```python
from build123d import *

# Parameters (mm, degrees)
BOSS_EXTRUDE1_DEPTH      = 48
BOSS_EXTRUDE2_DEPTH      = 107
BOSS_EXTRUDE2_DEPTH_BACK = 135
BOSS_EXTRUDE3_DEPTH      = 70


with BuildPart() as part:
    # Sketch6 → Boss-Extrude1 (new body)
    with BuildSketch(Plane.YZ):
        with BuildLine():
            Line((-18.5, 42), (9, 42))
            Line((9, 42), (9, -20))
            ThreePointArc((9, -20), (6.656854249, -25.656854249), (1, -28))
            Line((1, -28), (-10.5, -28))
            ThreePointArc((-10.5, -28), (-16.156854249, -25.656854249), (-18.5, -20))
            Line((-18.5, -20), (-18.5, 42))
        make_face()
    extrude(amount=-BOSS_EXTRUDE1_DEPTH)

    # Sketch7 → Boss-Extrude2 (add, two sides: drawn at the far end of the back side and taken through both)
    with BuildSketch(Plane.YZ.offset(-BOSS_EXTRUDE2_DEPTH_BACK)):
        with BuildLine():
            Line((6.7, 42), (6.7, 0))
            ThreePointArc((6.7, 0), (0, -6.7), (-6.7, 0))
            Line((-6.7, 0), (-6.7, 42))
            Line((-6.7, 42), (6.7, 42))
        make_face()
    extrude(amount=BOSS_EXTRUDE2_DEPTH + BOSS_EXTRUDE2_DEPTH_BACK)

    # Sketch8 → Boss-Extrude3 (add)
    with BuildSketch(Plane.YZ):
        with BuildLine():
            Line((-17.499999986, -6.99976205), (-19.468374717, 42))
            Line((-19.468374717, 42), (-11.531625283, 42))
            Line((-11.531625283, 42), (-13.500019034, -7.008725467))
            ThreePointArc((-13.500019034, -7.008725467), (-15.504481719, -8.999994979), (-17.499999986, -6.99976205))
        make_face()
    extrude(amount=BOSS_EXTRUDE3_DEPTH)

    # Loft2: read off the stored shape, not the designer's step
    # Loft2: loft between two sections, ruled curve by curve
    loft2_from = [
        Edge.make_bspline([(-43, -12.5, 42), (-43, -12.5, 36.250008881), (-43, -12.5, 24.641436529), (-43, -12.5, 7.145431099), (-43, -12.5, -10.177895331), (-43, -12.5, -21.457402798), (-43, -12.5, -27.496400477), (-43, -12.735353866, -28.366169962), (-43, -13.470979996, -29.306081404), (-43, -14.433479869, -29.873432167), (-43, -15.500002282, -30.063307511), (-43, -16.566524261, -29.873430596), (-43, -17.529022849, -29.306078761), (-43, -18.264647219, -28.36616736), (-43, -18.5, -27.496399176), (-43, -18.5, -21.457400197), (-43, -18.5, -10.177897954), (-43, -18.5, 7.145406937), (-43, -18.5, 24.641401673), (-43, -18.5, 36.249991119), (-43, -18.5, 42)], [0, 0, 0, 0, 0.114724944, 0.229449887, 0.344174831, 0.458899774, 0.458899774, 0.469174653, 0.479449533, 0.489724412, 0.499999291, 0.51027417, 0.52054905, 0.530823929, 0.541098808, 0.541098808, 0.655824106, 0.770549404, 0.885274702, 1, 1, 1, 1], 3),
        Edge.make_line((-43, -18.5, 42), (-43, -12.5, 42)),
    ]
    loft2_to = [
        Edge.make_bspline([(-90, -11.531625283, 42), (-90, -11.570656574, 37.916659954), (-90, -11.648004314, 29.824764413), (-90, -11.763499254, 17.742019914), (-90, -11.880008186, 5.553194479), (-90, -11.95947034, -2.759904881), (-90, -12, -7.379764452), (-90, -12.124025603, -8.182036975), (-90, -12.791211148, -9.362294599), (-90, -13.96862904, -10.268779081), (-90, -15.499994859, -10.616349391), (-90, -17.031362783, -10.268783245), (-90, -18.208784945, -9.362299724), (-90, -18.87597374, -8.182040057), (-90, -19, -7.379765435), (-90, -18.956733754, -2.759907847), (-90, -18.871906161, 5.553196207), (-90, -18.747530231, 17.742037363), (-90, -18.624236843, 29.824789377), (-90, -18.541666598, 37.916673379), (-90, -18.5, 42)], [0, 0, 0, 0, 0.114724944, 0.229449887, 0.344174831, 0.458899774, 0.458899774, 0.469174653, 0.479449533, 0.489724412, 0.499999291, 0.51027417, 0.52054905, 0.530823929, 0.541098808, 0.541098808, 0.655824106, 0.770549404, 0.885274702, 1, 1, 1, 1], 3),
        Edge.make_line((-90, -18.5, 42), (-90, -11.531625283, 42)),
    ]
    loft2 = Solid(Shell([*[Face.make_surface_from_curves(loft2_from[k], loft2_to[k]) for k in range(2)], Face(Wire(loft2_from)), Face(Wire(loft2_to))]))
    add(loft2)


solid = part.part
```
For this review, take the finished solid that the model builds, in its own axes (mm). A direction names the side the tool comes from. Coordinates: 2 decimals unless noted, no trailing zeros. Order: outer loops, then holes, each group sorted by start corner. A loop starts at its lowest first (then second) coordinate and runs counter-clockwise, first axis right, second up. Notation, with made-up numbers: (-26, 20) -> (1, 20) arc R30 ccw to (1, 59) -> close; hole circle Ø10 at (-34, 5). An arc over 180 degrees is marked (long way). Use CSV: the item, a comma, the result in double quotes. Start each with the question number.
Item 1: We need section A-A, the plane y = -3.25. Give the boundary of the cut face in (x, z), then the cut area to 3 significant figures.
Item 2: Wall thickness on probe 1 along Y at (x, z) = (1, 17); probe 2 along Y at (x, z) = (-110, 20); probe 3 along X at (y, z) = (-9.25, -4): over which ranges is each line inside the solid? List them lowest first.
Item 3: For faces 1 (the face through (0, -8, 0)), 2 (the face through (-92.1, 0.1, -6.7)), 3 (the face through (-90, -15, 16)), 4 (the face through (70, -15, 23)), 5 (the face through (34.51, -18.47, 17.16)), list the 3-axis set-ups (+Z, -Z, +X, -X, +Y, -Y) from which the entire face can be reached by the end or side of a thin tool; tool diameter is ignored.
Item 4: Draft analysis for pull direction Y (two halves, no side actions). For faces 6 (the face through (107, 0, 18)), 7 (the face through (53, 6.7, 21)), 8 (the face through (53, -6.7, 21)), state which applies: pulls with the +Y half, pulls with the -Y half, needs draft (parallel to the pull), parting line crosses it, or undercut.
Item 5: Insertion check: pin 1 (8 mm diameter, centred on x = -68, y = 2, fed in from -Z); pin 2 (2 mm diameter, centred on y = -15, z = 20, fed in from -X); pin 3 (12 mm diameter, centred on x = -93.5, z = 29, fed in from -Y). Each pin has a flat end and moves straight along its axis. Give the tip position at first contact, or say it passes through.
Derived:
1,outline,"(-135, -5.86) -> (-48, -5.86) -> (-48, -28) -> (0, -28) -> (0, -5.86) -> (107, -5.86) -> (107, 42) -> (-135, 42) -> close"
1,area,"12,600 mm^2"
2,probe 1,"y = -18.46 to -12.54, -6.7 to 6.7"
2,probe 2,"y = -6.7 to 6.7"
2,probe 3,"x = -48 to 0"
3,face 1,"-Z, +X"
3,face 2,"-Z, -X"
3,face 3,"+Z, -Z, -X, -Y"
3,face 4,"+Z, -Z, +X, -Y"
3,face 5,"-Z, +X, -Y"
4,face 6,"needs draft"
4,face 7,"pulls with the +Y half"
4,face 8,"undercut"
5,pin 1,"stops at z = -6.7"
5,pin 2,"stops at x = -90"
5,pin 3,"stops at y = -18.68"
